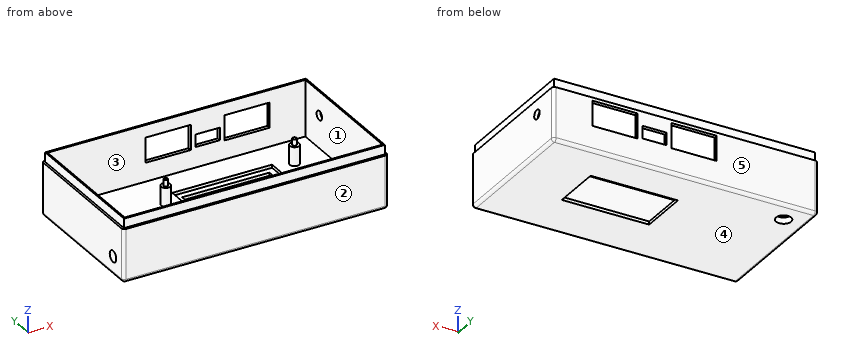
```python
from build123d import *

# Parameters (mm, degrees)
SKETCH_1_W          = 85
SKETCH_1_H          = 45
EXTRUDE_1_DEPTH     = 20
SKETCH_2_W          = 82.6
SKETCH_2_H          = 42.6
CUT_EXTRUDE_1_DEPTH = 18
SKETCH_3_R          = 52.564832307
SKETCH_3_W          = 83.6
SKETCH_3_H          = 43.6
CUT_EXTRUDE_2_DEPTH = 3
SKETCH_4_R          = 1.5
CUT_EXTRUDE_3_DEPTH = 10
SKETCH_6_R          = 1.5
EXTRUDE_2_DEPTH     = 6
SKETCH_7_R          = 0.65
EXTRUDE_3_DEPTH     = 2
SKETCH_5_W          = 28
SKETCH_5_H          = 15.9
CUT_EXTRUDE_4_DEPTH = 99.234413522
SKETCH_9_W          = 32
SKETCH_9_H          = 19.9
CUT_EXTRUDE_5_DEPTH = 1
SKETCH_10_W         = 14.5
SKETCH_10_H         = 8
SKETCH_10_W_2       = 7.8
SKETCH_10_H_2       = 4
CUT_EXTRUDE_6_DEPTH = 10
FILLET_1_R          = 1
SKETCH_11_R         = 1.8
EXTRUDE_4_DEPTH     = 10
SKETCH_12_R         = 1.8
CUT_EXTRUDE_7_DEPTH = 90.721792225
SKETCH_13_R         = 2.425
CUT_EXTRUDE_8_DEPTH = 98.846819059


with BuildPart() as part:
    # Эскиз1 → Бобышка-Вытянуть1 (new body)
    with BuildSketch(Plane.XY):
        with Locations((42.5, 22.5)):
            Rectangle(SKETCH_1_W, SKETCH_1_H)
    extrude(amount=EXTRUDE_1_DEPTH)

    # Эскиз2 → Вырез-Вытянуть1 (cut)
    with BuildSketch(Plane.XY.offset(20)):
        with Locations((42.5, 22.5)):
            Rectangle(SKETCH_2_W, SKETCH_2_H)
    extrude(amount=-CUT_EXTRUDE_1_DEPTH, mode=Mode.SUBTRACT)

    # Эскиз3 → Вырез-Вытянуть2 (cut)
    with BuildSketch(Plane.XY.offset(20)):
        with Locations((42.5, 22.5)):
            Circle(SKETCH_3_R)
        with Locations((42.5, 22.5)):
            Rectangle(SKETCH_3_W, SKETCH_3_H, mode=Mode.SUBTRACT)
    extrude(amount=-CUT_EXTRUDE_2_DEPTH, mode=Mode.SUBTRACT)

    # Эскиз4 → Вырез-Вытянуть3 (cut)
    with BuildSketch(Plane.ZY.offset(-85)):
        with Locations(Location((12.4, 36.05, 0), (0, 0, 180))):
            Circle(SKETCH_4_R)
    extrude(amount=CUT_EXTRUDE_3_DEPTH, mode=Mode.SUBTRACT)

    # Эскиз6 → Бобышка-Вытянуть2 (add)
    with BuildSketch(Plane.XY.offset(2)):
        with Locations((31, 29.89)):
            Circle(SKETCH_6_R)
        with Locations((73.5, 32)):
            Circle(SKETCH_6_R)
    extrude(amount=EXTRUDE_2_DEPTH)

    # Эскиз7 → Бобышка-Вытянуть3 (add)
    with BuildSketch(Plane.XY.offset(8)):
        with Locations((31, 29.89)):
            Circle(SKETCH_7_R)
        with Locations((73.5, 32)):
            Circle(SKETCH_7_R)
    extrude(amount=EXTRUDE_3_DEPTH)

    # Эскиз5 → Вырез-Вытянуть4 (cut, through all)
    with BuildSketch(Plane(origin=(0, 0, 0), x_dir=(-1, 0, 0), z_dir=(0, 0, -1))):
        with Locations((-51.8, 24.64)):
            Rectangle(SKETCH_5_W, SKETCH_5_H)
    extrude(amount=-CUT_EXTRUDE_4_DEPTH, mode=Mode.SUBTRACT)

    # Эскиз9 → Вырез-Вытянуть5 (cut)
    with BuildSketch(Plane.XY.offset(2)):
        with Locations((51.8, 24.64)):
            Rectangle(SKETCH_9_W, SKETCH_9_H)
    extrude(amount=-CUT_EXTRUDE_5_DEPTH, mode=Mode.SUBTRACT)

    # Эскиз10 → Вырез-Вытянуть6 (cut)
    with BuildSketch(Plane.XZ.offset(-45)):
        with Locations((39.85, 12)):
            Rectangle(SKETCH_10_W, SKETCH_10_H)
        with Locations((65.15, 12)):
            Rectangle(SKETCH_10_W, SKETCH_10_H)
        with Locations((52.5, 10.5)):
            Rectangle(SKETCH_10_W_2, SKETCH_10_H_2)
    extrude(amount=CUT_EXTRUDE_6_DEPTH, mode=Mode.SUBTRACT)

    # Скругление1
    fillet_1_edges = [part.edges().sort_by_distance(p)[0] for p in [
        (0, 45, 8.5),
        (85, 45, 8.5),
        (85, 0, 8.5),
        (0, 0, 8.5),
        (42.5, 45, 0),
        (85, 22.5, 0),
        (42.5, 0, 0),
        (0, 22.5, 0),
    ]]
    fillet(fillet_1_edges, radius=FILLET_1_R)

    # Эскиз11 → Бобышка-Вытянуть4 (add)
    with BuildSketch(Plane.ZY):
        with BuildLine():
            Line((1, 7.094213846), (1, 4.094213846))
            Line((1, 4.094213846), (4.208818791, 3.094213846))
            ThreePointArc((4.208818791, 3.094213846), (8.867131186, 5.594213846), (4.208818791, 8.094213846))
            Line((4.208818791, 8.094213846), (1, 7.094213846))
        make_face()
        with Locations((5.867131186, 5.594213846)):
            Circle(SKETCH_11_R, mode=Mode.SUBTRACT)
    extrude(amount=-EXTRUDE_4_DEPTH)

    # Эскиз12 → Вырез-Вытянуть7 (cut, through all)
    with BuildSketch(Plane(origin=(10, 0, 0), x_dir=(0, 0, -1), z_dir=(1, 0, 0))):
        with Locations(Location((-5.867131186, 5.594213846, 0), (0, 0, 180))):
            Circle(SKETCH_12_R)
    extrude(amount=-CUT_EXTRUDE_7_DEPTH, mode=Mode.SUBTRACT)

    # Эскиз13 → Вырез-Вытянуть8 (cut, through all)
    with BuildSketch(Plane.XY.offset(2)):
        with Locations((7, 37.89)):
            Circle(SKETCH_13_R)
    extrude(amount=-CUT_EXTRUDE_8_DEPTH, mode=Mode.SUBTRACT)


solid = part.part
```
Check sheet for the modelled part. Datum: model origin and axes. Units: mm. Face numbers are marked on the shaded views. A direction names the side the tool comes from. Give positions to 0.01 mm unless a question says otherwise; leave off trailing zeros. Order: outer loops, then holes, each group sorted by start corner. A loop starts at its lowest first (then second) coordinate and runs counter-clockwise, first axis right, second up. Notation, with made-up numbers: M 48,-28 L 71,-28 A21 cw 71,-24 Z; hole C -11,10.25 d9. An arc over 180 degrees is marked long. Answer in a Markdown table with one row per item. Add a question column.
Q1. Release check for a two-part mould opening along Y. For the marked faces 3, 4 and 5 record: released by +Y, released by -Y, zero draft, split by the parting line, or undercut.
Q2. Sectioned sample at D-D, the plane x = 28. Record the boundary of the cut face in (y, z).
Q3. Sectioned sample at B-B, the plane y = 22.5. Record the boundary of the cut face in (x, z), and give its area (3 significant figures).
Q4. Thickness scan on L1, parallel to X at y = 13.5, z = 8.25; L2, parallel to Y at x = 7, z = 1.5 (3 decimals); L3, parallel to Z at x = 84, y = 36. Record the ranges inside material, lowest first.
Q5. Sectioned sample at A-A, the plane x = 7. Record the boundary of the cut face in (y, z) (3 decimals), and give its area (3 significant figures).
Q6. Sectioned sample at C-C, the plane x = 62. Record the boundary of the cut face in (y, z).
Q7. Access from +Z, -Z, +X, -X, +Y, -Y to the whole of each face (thin tool, end or side, straight path). Record for the marked faces 1 and 2.
Q8. Gauge pin test, flat ends, axial feed: pin 1 Ø1.5 at (y, z) = (26.5, 18.5) entering from +X; pin 2 Ø0.8 at (y, z) = (21, 0.5) entering from +X (3 decimals); pin 3 Ø1 at (x, y) = (73.5, 32) entering from +Z; pin 4 Ø3 at (x, y) = (7, 37.89) entering from -Z. Record the tip position at first contact, or that the pin passes through.
Verdict:
| question | item | result |
|---|---|---|
| 1 | face 3 | undercut |
| 1 | face 4 | zero draft |
| 1 | face 5 | released by +Y |
| 2 | outline | M 0,1 A1 ccw 1,0 L 44,0 A1 ccw 45,1 L 45,17 L 44.3,17 L 44.3,20 L 43.8,20 L 43.8,2 L 1.2,2 L 1.2,20 L 0.7,20 L 0.7,17 L 0,17 Z |
| 3 | outline | M 0,1 A1 ccw 1,0 L 37.8,0 L 37.8,1 L 35.8,1 L 35.8,2 L 1.2,2 L 1.2,20 L 0.7,20 L 0.7,17 L 0,17 Z; M 65.8,0 L 84,0 A1 ccw 85,1 L 85,17 L 84.3,17 L 84.3,20 L 83.8,20 L 83.8,2 L 67.8,2 L 67.8,1 L 65.8,1 Z |
| 3 | area | 149 mm² |
| 4 | L1 | 0 to 1.2, 83.8 to 85 |
| 4 | L2 | 0 to 35.465, 40.315 to 45 |
| 4 | L3 | 0 to 10.9, 13.9 to 20 |
| 5 | outline | M 0,1 A1 ccw 1,0 L 35.465,0 L 35.465,2 L 7.406,2 L 8.094,4.209 A3 ccw long 3.094,4.209 L 3.783,2 L 1.2,2 L 1.2,20 L 0.7,20 L 0.7,17 L 0,17 Z; M 40.315,0 L 44,0 A1 ccw 45,1 L 45,17 L 44.3,17 L 44.3,20 L 43.8,20 L 43.8,2 L 40.315,2 Z; hole C 5.594,5.867 d3.6 |
| 5 | area | 142 mm² |
| 6 | outline | M 0,1 A1 ccw 1,0 L 16.69,0 L 16.69,1 L 14.69,1 L 14.69,2 L 1.2,2 L 1.2,20 L 0.7,20 L 0.7,17 L 0,17 Z; M 32.59,0 L 44,0 A1 ccw 45,1 L 45,8 L 43.8,8 L 43.8,2 L 34.59,2 L 34.59,1 L 32.59,1 Z; M 43.8,16 L 45,16 L 45,17 L 44.3,17 L 44.3,20 L 43.8,20 Z |
| 7 | face 1 | +Z |
| 7 | face 2 | +Z, -Z, +X, -X, -Y |
| 8 | pin 1 | x = 84.3 |
| 8 | pin 2 | x = 84.995 |
| 8 | pin 3 | z = 10 |
| 8 | pin 4 | through |
